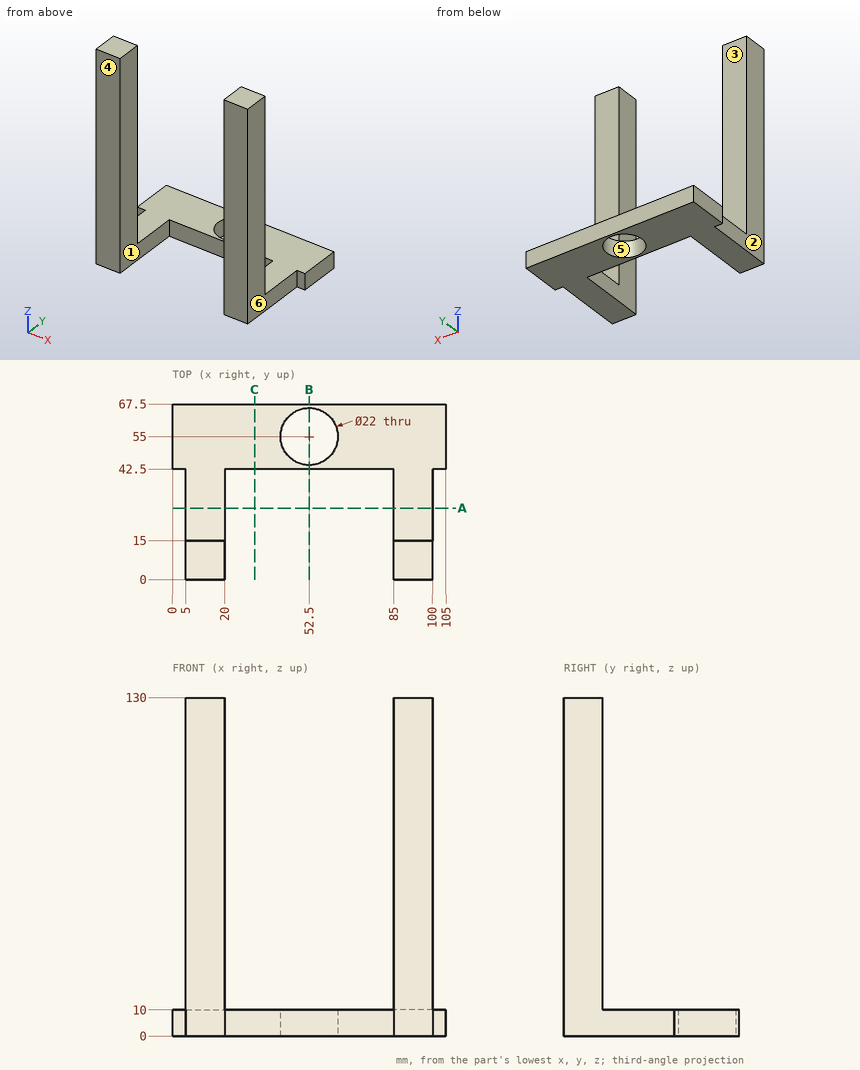
For this review, use the dimensioned drawing (mm, ordinates from the lowest corner) and the shaded views. A direction names the side the tool comes from. Round coordinates to 2 decimals unless told otherwise and drop trailing zeros. Order: outer loops, then holes, each group sorted by start corner. A loop starts at its lowest first (then second) coordinate and runs counter-clockwise, first axis right, second up. Notation, with made-up numbers: (3, 34.25) - (19, 34.25) arc R18 cw to (19, 39.25) - close; hole circle Ø8 at (43, 37). An arc over 180 degrees is marked (long way). Use one line per item in the form item = value.
Q1. Add section C-C on x = 31.5. Give the boundary of the cut face in (y, z).
Response values:
outline = (42.5, 0) - (67.5, 0) - (67.5, 10) - (42.5, 10) - close
Q2. Clearance check with flat-ended pins moving along their axes: P1, Ø4, axis at x = 103, z = 7, coming from the -Y side; P2, Ø7.5, axis at x = 13.5, z = 78.5, coming from the +Y side. State where each tip first meets the part, or that it passes through.
Response values:
P1 = 42.5
P2 = 15
Q3. Add section A-A on y = 27.5. Give the boundary of the cut face in (x, z), then the cut area to 3 significant figures.
Response values:
outline = (5, 0) - (20, 0) - (20, 10) - (5, 10) - close; (85, 0) - (100, 0) - (100, 10) - (85, 10) - close
area = 300 mm^2
Q4. To check wall thickness, follow line 1 (X direction, y = 13, z = 95.5); line 2 (Y direction, x = 52.5, z = 3.5); line 3 (Z direction, x = 96.5, y = 47). State the ranges of each line that lie inside material, in increasing order.
Response values:
line_1 = 5 to 20, 85 to 100
line_2 = 42.5 to 44, 66 to 67.5
line_3 = 0 to 10
Q5. Add section B-B on x = 52.5. Give the boundary of the cut face in (y, z).
Response values:
outline = (42.5, 0) - (44, 0) - (44, 10) - (42.5, 10) - close; (66, 0) - (67.5, 0) - (67.5, 10) - (66, 10) - close
Q6. Tool access review of the marked faces 1, 2 and 3: name each direction out of +Z, -Z, +X, -X, +Y, -Y from which nothing blocks a thin tool from reaching the whole face with its end or side.
Response values:
face_1 = +Z, -Z, -Y
face_2 = +Z, -Z, -X, -Y
face_3 = +Z, +X, -X, +Y
Q7. Mouldability with a two-part tool opening along X and no side actions: class the marked faces 4, 5 and 6 as pulls with the +X half, pulls with the -X half, needs draft (parallel to the pull), parting line crosses it, or undercut.
Response values:
face_4 = needs draft
face_5 = undercut
face_6 = pulls with the +X half
